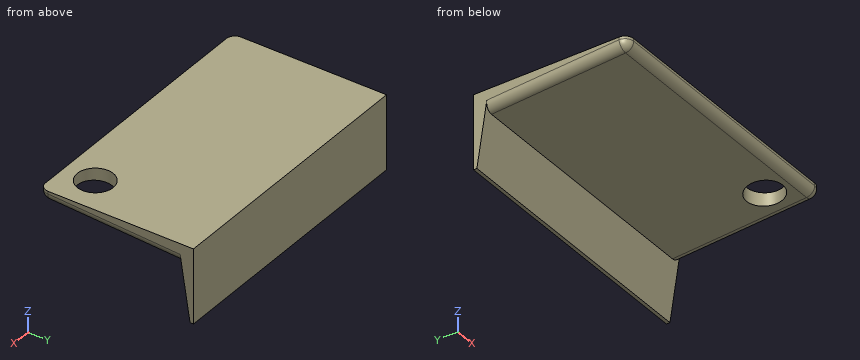
from build123d import *

# Parameters (mm, degrees)
F1_DEPTH = 80
F2_R     = 10.5
F3_DEPTH = 25
F4_R     = 5


with BuildPart() as f1:
    # F0 (on Right) → F1 (new body, symmetric)
    with BuildSketch(Plane.YZ):
        Polygon((55.125829, 22.787926), (-34.874171, 22.787926), (-34.874171, 16.537924), (48.125829, 11.537924), (53.125829, -20.545409), (55.125829, -20.545409), align=None)
    extrude(amount=F1_DEPTH, both=True)

    # F2 (on face) → F3 (cut)
    with BuildSketch(Plane.XY.offset(22.787926)):
        with Locations((59.5, -16.65573)):
            Circle(F2_R)
    extrude(amount=-F3_DEPTH, mode=Mode.SUBTRACT)

    # F4
    f4_edges = [f1.edges().sort_by_distance(p)[0] for p in [
        (80, -34.874171, 19.662925),
        (-80, -34.874171, 19.662925),
        (80, 6.625829, 14.037924),
        (-80, 6.625829, 14.037924),
        (0, -34.874171, 16.537924),
    ]]
    fillet(f4_edges, radius=F4_R)


solid = f1.part
Input: part model. Units: mm. Frame: model coordinates. Coordinates: 2 decimals unless noted, no trailing zeros. Loops run counter-clockwise (first coordinate to the right, second up) from the corner with the lowest first, then second, coordinate; pieces in that order, holes last.
Q1. Cut plane C-C (z = 8.5). Output: boundary loops of the cut face in (x, y).
Q2. Cut plane D-D (z = -12). Output: boundary loops of the cut face in (x, y), then the cut area to 3 significant figures.
Q3. Contact query for flat-ended pins moving along their axis: pin 1 (8 mm diameter, centred on x = 46.5, y = -16.5, fed in from -Z); pin 2 (10 mm diameter, centred on x = -1.5, y = -10.5, fed in from -Z); pin 3 (24 mm diameter, centred on x = 59.5, y = -16.66, fed in from +Z); pin 4 (10 mm diameter, centred on x = 13, z = -12.5, fed in from -Y). Output: stop coordinate, or through.
Q4. Material intervals for line 1 (Y direction, x = 59, z = 19); line 2 (Y direction, x = 59, z = 20); line 3 (Y direction, x = 72.5, z = -4.5), sorted ascending.
Q5. Cut plane A-A (x = 2.5). Output: boundary loops of the cut face in (y, z), then the cut area to 3 significant figures.
Q6. Cut plane B-B (x = 59.5). Output: boundary loops of the cut face in (y, z).
Working result:
1. outline: (-80, 48.6) - (80, 48.6) - (80, 55.13) - (-80, 55.13) - close
2. outline: (-80, 51.79) - (80, 51.79) - (80, 55.13) - (-80, 55.13) - close
2. area: 533 mm2
3. pin 1: stops at z = 15.19
3. pin 2: stops at z = 14.77
3. pin 3: stops at z = 22.79
3. pin 4: stops at y = 51.09
4. line 1: y = -34.34 to -27.14, -6.17 to 55.13
4. line 2: y = -34.72 to -27.14, -6.17 to 55.13
4. line 3: y = 50.63 to 55.13
5. outline: (-34.87, 21.25) arc R5 ccw to (-30.17, 16.25) - (48.13, 11.54) - (53.13, -20.55) - (55.13, -20.55) - (55.13, 22.79) - (-34.87, 22.79) - close
5. area: 945 mm2
6. outline: (-34.87, 21.25) arc R5 ccw to (-30.17, 16.25) - (-27.16, 16.07) - (-27.16, 22.79) - (-34.87, 22.79) - close; (-6.16, 14.81) - (48.13, 11.54) - (53.13, -20.55) - (55.13, -20.55) - (55.13, 22.79) - (-6.16, 22.79) - close
